```python
from build123d import *

# Parameters (mm, degrees)
SKETCH1_W           = 150
SKETCH1_H           = 65
BOSS_EXTRUDE1_DEPTH = 40
SKETCH2_W           = 143.904
SKETCH2_H           = 58.904
CUT_EXTRUDE1_DEPTH  = 28.4
SKETCH3_R           = 4
CUT_EXTRUDE2_DEPTH  = 3.048


with BuildPart() as part:
    # Sketch1 → Boss-Extrude1 (new body)
    with BuildSketch(Plane(origin=(0, 0, 0), x_dir=(1, 0, 0), z_dir=(0, 1, 0))):
        Rectangle(SKETCH1_W, SKETCH1_H)
    extrude(amount=BOSS_EXTRUDE1_DEPTH)

    # Sketch2 → Cut-Extrude1 (cut)
    with BuildSketch(Plane.XZ):
        Rectangle(SKETCH2_W, SKETCH2_H)
    extrude(amount=-CUT_EXTRUDE1_DEPTH, mode=Mode.SUBTRACT)

    # Sketch3 → Cut-Extrude2 (cut)
    with BuildSketch(Plane(origin=(0, 0, -32.5), x_dir=(-1, 0, 0), z_dir=(0, 0, -1))):
        with Locations((38.12, 12.19)):
            Circle(SKETCH3_R)
    extrude(amount=-CUT_EXTRUDE2_DEPTH, mode=Mode.SUBTRACT)


solid = part.part
```
Input: part model. Units: mm. Frame: model coordinates. A direction names the side the tool comes from. Round coordinates to 2 decimals unless told otherwise and drop trailing zeros. Loops run counter-clockwise (first coordinate to the right, second up) from the corner with the lowest first, then second, coordinate; pieces in that order, holes last.
1) Section query A-A on x = -38.12. Return the cut outline in (y, z), plus the area to 3 significant figures.
Ans:
outline: (0, -32.5) - (8.19, -32.5) - (8.19, -29.45) - (0, -29.45) - close; (0, 29.45) - (28.4, 29.45) - (28.4, -29.45) - (16.19, -29.45) - (16.19, -32.5) - (40, -32.5) - (40, 32.5) - (0, 32.5) - close
area: 903 mm2
2) Pull-direction query (X, two-part tool) for faces 4 (the flat face through (-1, 14, -29.452)), 5 (the flat face through (75, 20, 0)), 6 (the flat face through (-1, 20, -32.5)); classes: released by +X, released by -X, zero draft, split by the parting line, or undercut.
Ans:
face 4: undercut
face 5: released by +X
face 6: zero draft
3) Section query B-B on y = 12.19. Return the cut outline in (x, z), plus the area to 3 significant figures.
Ans:
outline: (-75, -32.5) - (-42.12, -32.5) - (-42.12, -29.45) - (-71.95, -29.45) - (-71.95, 29.45) - (71.95, 29.45) - (71.95, -29.45) - (-34.12, -29.45) - (-34.12, -32.5) - (75, -32.5) - (75, 32.5) - (-75, 32.5) - close
area: 1,250 mm2
4) Section query D-D on x = 47. Return the cut outline in (y, z).
Ans:
outline: (0, -32.5) - (40, -32.5) - (40, 32.5) - (0, 32.5) - (0, 29.45) - (28.4, 29.45) - (28.4, -29.45) - (0, -29.45) - close
5) Set-up query: faces 1 (the flat face through (-23, 0, -31)), 2 (the cylindrical face through (-34.124, 12.366, -30.997)), 3 (the flat face through (-1, 14, 29.452)). Return all of +Z, -Z, +X, -X, +Y, -Y with unobstructed straight access to the full face (end or side cutting, diameter ignored); none if empty.
Ans:
face 1: +Z, -Z, +X, -X, -Y
face 2: -Z
face 3: -Y
6) Section query C-C on z = -9.5. Return the cut outline in (x, y).
Ans:
outline: (-75, 0) - (-71.95, 0) - (-71.95, 28.4) - (71.95, 28.4) - (71.95, 0) - (75, 0) - (75, 40) - (-75, 40) - close
7) Material intervals for line 1 (X direction, y = 23, z = 4); line 2 (Y direction, x = -38, z = -30); line 3 (Z direction, x = -53, y = 18.5), sorted ascending.
Ans:
line 1: x = -75 to -71.95, 71.95 to 75
line 2: y = 0 to 8.19, 16.19 to 40
line 3: z = -32.5 to -29.45, 29.45 to 32.5
